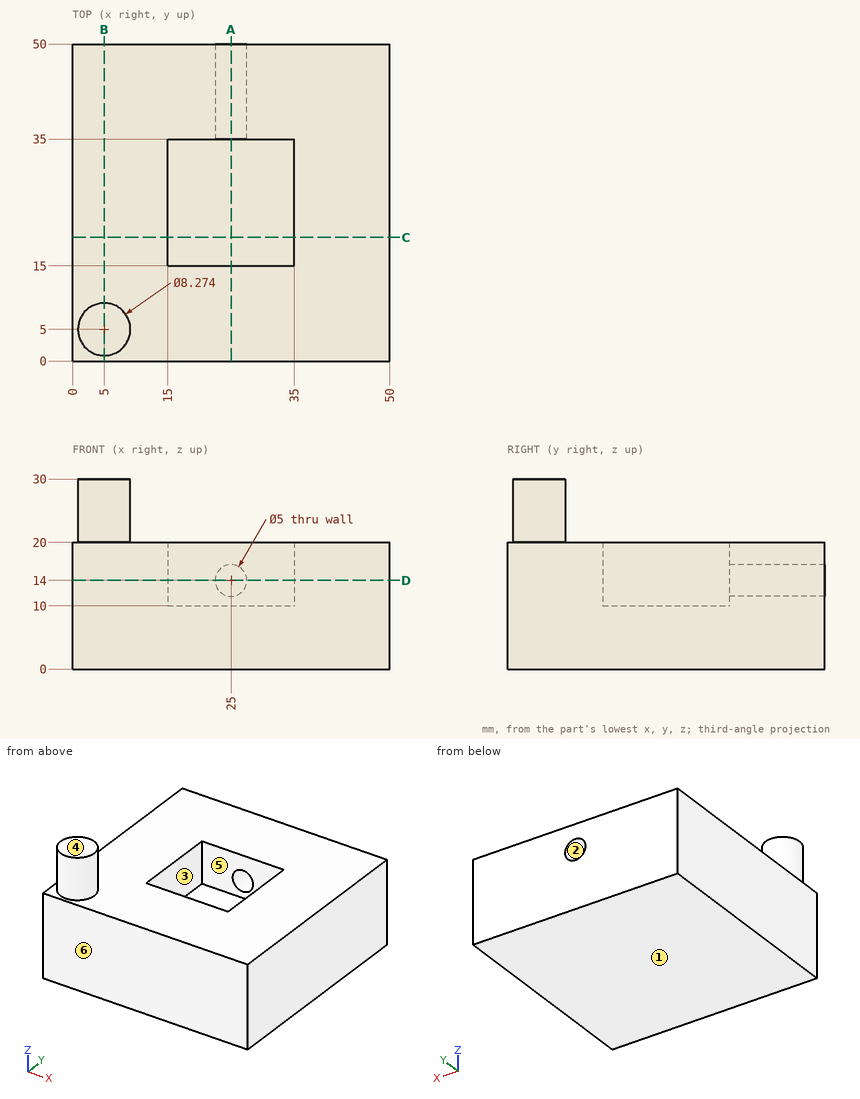
Answer from the drawing. Dimensions are ordinates in mm from the lowest x, y and z of the part. A direction names the side the tool comes from. Give positions to 0.01 mm unless a question says otherwise; leave off trailing zeros. Loops run counter-clockwise (first coordinate to the right, second up) from the corner with the lowest first, then second, coordinate; pieces in that order, holes last. Notation, with made-up numbers: (3.5, 38) -> (28.5, 38) arc R14 cw to (28.5, 59) -> close; hole circle Ø6 at (79.25, 69). An arc over 180 degrees is marked (long way). One line per question, with ' | ' between items. Start each with the question number.
1) Each of these flat-tipped pins is pushed along its axis until it touches: pin 1 (15 mm diameter, centred on x = 32, y = 13.5, fed in from +Z); pin 2 (8 mm diameter, centred on x = 6.5, y = 38.5, fed in from -Z); pin 3 (6 mm diameter, centred on x = 26, y = 24.5, fed in from +Z). Where does it stop, or does it pass through?
2) Determine the mould class of the marked faces 4, 5 and 6 for opening direction Y: +Y half, -Y half, draft (parallel to the pull), parting line (faces both ways), or undercut.
3) Section C-C, the plane y = 19.5 is taken. Determine the outline of the cut face in (x, z).
4) Section D-D, the plane z = 14 is taken. Determine the outline of the cut face in (x, y).
5) Section A-A, the plane x = 25 is taken. Determine the outline of the cut face in (y, z), then the cut area to 3 significant figures.
6) Section B-B, the plane x = 5 is taken. Determine the outline of the cut face in (y, z), then the cut area to 3 significant figures.
7) Straight lines are drawn through the part: L1, parallel to X at y = 26, z = 16.5; L2, parallel to Z at x = 25, y = 39.25. For each, find the intervals that lie inside material, in ascending order.
8) For the marked faces 1, 2 and 3, determine the directions among +Z, -Z, +X, -X, +Y, -Y from which every point of the face is accessible in a straight line to the end or side of a thin tool.
Resolved:
1) pin 1: z = 20 | pin 2: z = 0 | pin 3: z = 10
2) face 4: draft | face 5: undercut | face 6: -Y half
3) outline: (0, 0) -> (50, 0) -> (50, 20) -> (35, 20) -> (35, 10) -> (15, 10) -> (15, 20) -> (0, 20) -> close
4) outline: (0, 0) -> (50, 0) -> (50, 50) -> (27.5, 50) -> (27.5, 35) -> (35, 35) -> (35, 15) -> (15, 15) -> (15, 35) -> (22.5, 35) -> (22.5, 50) -> (0, 50) -> close
5) outline: (0, 0) -> (50, 0) -> (50, 11.5) -> (35, 11.5) -> (35, 10) -> (15, 10) -> (15, 20) -> (0, 20) -> close; (35, 16.5) -> (50, 16.5) -> (50, 20) -> (35, 20) -> close | area: 725 mm2
6) outline: (0, 0) -> (50, 0) -> (50, 20) -> (9.14, 20) -> (9.14, 30) -> (0.86, 30) -> (0.86, 20) -> (0, 20) -> close | area: 1,080 mm2
7) L1: 0 to 15, 35 to 50 | L2: 0 to 11.5, 16.5 to 20
8) face 1: -Z, +X, -X, +Y, -Y | face 2: +Y | face 3: +Z
